Design review of the part built by this model. Coordinates are the model's own, in mm. Round coordinates to 2 decimals unless told otherwise and drop trailing zeros. Loops run counter-clockwise (first coordinate to the right, second up) from the corner with the lowest first, then second, coordinate; pieces in that order, holes last. Notation, with made-up numbers: (55, 68) - (95, 68) arc R27 ccw to (95, 93) - close; hole circle Ø11 at (-28.75, -24). An arc over 180 degrees is marked (long way). Use one line per item in the form item = value. Start each with the question number.
(1) We need section C-C, the plane z = 3.75. Give the number of separate pieces and of enclosed holes in the cut face, then the cut area to 3 significant figures.
(2) Wall thickness on probe 1 along Y at (x, z) = (82.5, 4); probe 2 along Y at (x, z) = (12, 5.5); probe 3 along X at (y, z) = (71, 3.5): over which ranges is each line inside the solid? List them lowest first. Write a range as [from, to].
(3) The part is to be moulded in two halves that separate along Y. For faces 1 (the cylindrical face through (63.081, 7.735, 5.07)), 2 (the cylindrical face through (147.15, 106.99, 4.93)), 3 (the flat face through (-150, 1, 5)), 4 (the cylindrical face through (23.081, 9.735, 5.07)), say which applies: released by +Y, released by -Y, zero draft, split by the parting line, or undercut.
(4) We need section B-B, the plane y = 71. Write out the cut boundary in (x, z), then the cut area to 3 significant figures.
(5) We need section A-A, the plane x = -15. Write out the cut boundary in (y, z).
from build123d import *

# Parameters (mm, degrees)
F1_DEPTH = 10
F2_R     = 10
F2_R_2   = 15
F3_DEPTH = 10


with BuildPart() as f1:
    # F0 (on Top) → F1 (new body)
    with BuildSketch(Plane.XY):
        with BuildLine():
            Line((140, 110), (-140, 110))
            ThreePointArc((-140, 110), (-147.071068, 107.071068), (-150, 100))
            Line((-150, 100), (-150, -100))
            ThreePointArc((-150, -100), (-147.071068, -107.071068), (-140, -110))
            Line((-140, -110), (140, -110))
            ThreePointArc((140, -110), (147.071068, -107.071068), (150, -100))
            Line((150, -100), (150, 100))
            ThreePointArc((150, 100), (147.071068, 107.071068), (140, 110))
        make_face()
    extrude(amount=F1_DEPTH)

    # F2 (on face) → F3 (cut)
    with BuildSketch(Plane.XY.offset(10)):
        with Locations((-83.84011, 16.042637)):
            Circle(F2_R)
        with Locations((-18.84011, 41.042637)):
            Circle(F2_R_2)
        with Locations((16.15989, 63.042637)):
            Circle(F2_R_2)
        with Locations((56.15989, 61.042637)):
            Circle(F2_R_2)
        with Locations((96.15989, 59.042637)):
            Circle(F2_R_2)
        with Locations((96.15989, 19.042637)):
            Circle(F2_R_2)
        with Locations((56.15989, 21.042637)):
            Circle(F2_R_2)
        with Locations((16.15989, 23.042637)):
            Circle(F2_R_2)
        with Locations((-18.84011, 1.042637)):
            Circle(F2_R_2)
    extrude(amount=-F3_DEPTH, mode=Mode.SUBTRACT)


solid = f1.part
Data:
q1.separate_pieces = 1
q1.enclosed_holes = 9
q1.area = 59,900 mm^2
q2.probe_1 = [-110, 12.85], [25.24, 52.85], [65.24, 110]
q2.probe_2 = [-110, 8.63], [37.45, 48.63], [77.45, 110]
q2.probe_3 = [-150, 3.44], [28.88, 44.94], [67.38, 87.1], [105.22, 150]
q3.face_1 = undercut
q3.face_2 = released by +Y
q3.face_3 = zero draft
q3.face_4 = undercut
q4.outline = (-150, 0) - (3.44, 0) - (3.44, 10) - (-150, 10) - close; (28.88, 0) - (44.94, 0) - (44.94, 10) - (28.88, 10) - close; (67.38, 0) - (87.1, 0) - (87.1, 10) - (67.38, 10) - close; (105.22, 0) - (150, 0) - (150, 10) - (105.22, 10) - close
q4.area = 2,340 mm^2
q5.outline = (-110, 0) - (-13.46, 0) - (-13.46, 10) - (-110, 10) - close; (15.54, 0) - (26.54, 0) - (26.54, 10) - (15.54, 10) - close; (55.54, 0) - (110, 0) - (110, 10) - (55.54, 10) - close
